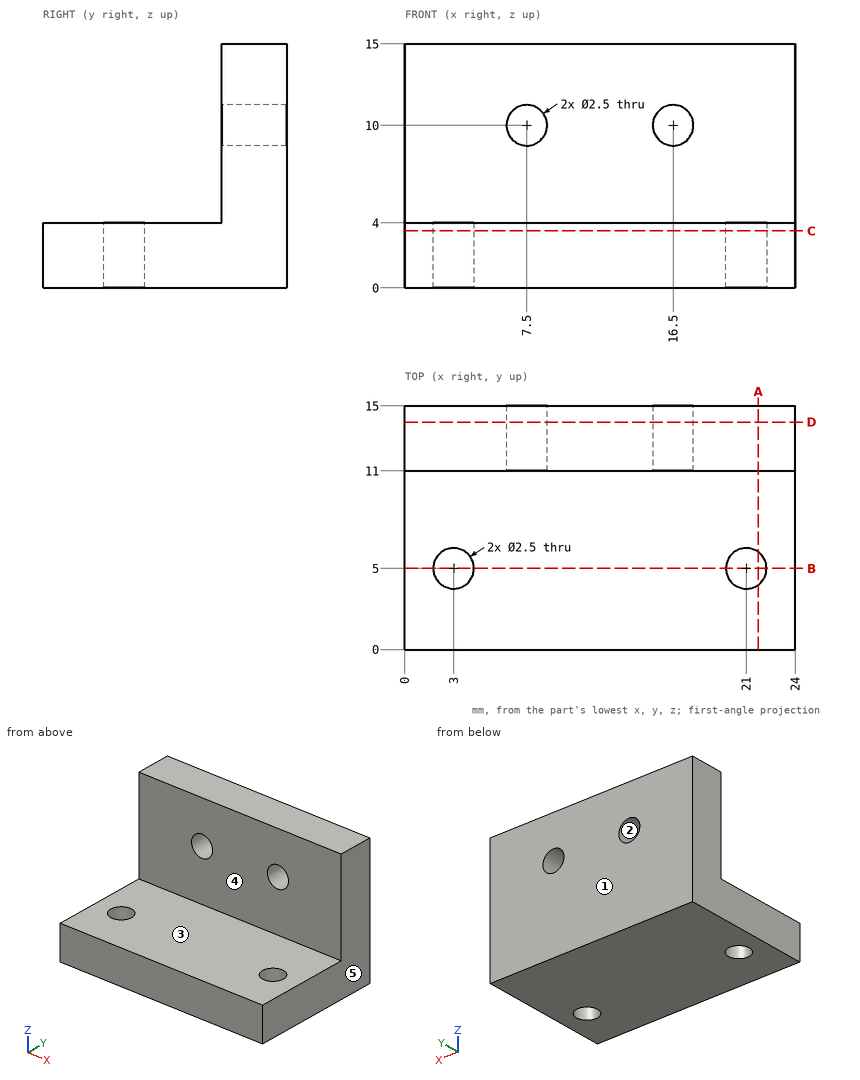
Answer from the drawing. Dimensions are ordinates in mm from the lowest x, y and z of the part. A direction names the side the tool comes from. Round coordinates to 2 decimals unless told otherwise and drop trailing zeros. Loops run counter-clockwise (first coordinate to the right, second up) from the corner with the lowest first, then second, coordinate; pieces in that order, holes last. Notation, with made-up numbers: (36.25, -24) - (68.25, -24) arc R9 ccw to (68.25, -19) - close; hole circle Ø9 at (68, 83). An arc over 180 degrees is marked (long way). Return JSON: item names as keys, results as strings. Group by question number.
1. The part is cut by section D-D on y = 14. Determine the outline of the cut face in (x, z).
2. The part is cut by section B-B on y = 5. Determine the outline of the cut face in (x, z), then the cut area to 3 significant figures.
3. Consider probe 1 along Z at (x, y) = (16.5, 13.4); probe 2 along Y at (x, z) = (21, 2.9); probe 3 along Y at (x, z) = (7.25, 7.5). Determine where each line is inside the solid, lowest interval first.
4. The part is cut by section C-C on z = 3.5. Determine the outline of the cut face in (x, y).
5. The part is cut by section A-A on x = 21.75. Determine the outline of the cut face in (y, z), then the cut area to 3 significant figures.
6. Which of the six approach directions +Z, -Z, +X, -X, +Y, -Y give full straight-line access (tool end or side, diameter ignored) to the marked faces 4 and 5?
7. Each of these flat-tipped pins is pushed along its axis until it touches: P1, Ø5.5, axis at x = 14.5, y = 4.5, coming from the +Z side; P2, Ø4, axis at x = 16.5, z = 10, coming from the -Y side. Where does it stop, or does it pass through?
8. The mould has two halves that part along Z. Classify the marked faces 1, 2 and 3: pulls with the +Z half, pulls with the -Z half, needs draft (parallel to the pull), parting line crosses it, or undercut.
Resolved:
{
 "1": {"outline": "(0, 0) - (24, 0) - (24, 15) - (0, 15) - close; hole circle Ø2.5 at (7.5, 10); hole circle Ø2.5 at (16.5, 10)"},
 "2": {"outline": "(0, 0) - (1.75, 0) - (1.75, 4) - (0, 4) - close; (4.25, 0) - (19.75, 0) - (19.75, 4) - (4.25, 4) - close; (22.25, 0) - (24, 0) - (24, 4) - (22.25, 4) - close", "area": "76.0 mm²"},
 "3": {"probe 1": "z = 0 to 8.75, 11.25 to 15", "probe 2": "y = 0 to 3.75, 6.25 to 15", "probe 3": "y = 11 to 15"},
 "4": {"outline": "(0, 0) - (24, 0) - (24, 15) - (0, 15) - close; hole circle Ø2.5 at (3, 5); hole circle Ø2.5 at (21, 5)"},
 "5": {"outline": "(0, 0) - (4, 0) - (4, 4) - (0, 4) - close; (6, 0) - (15, 0) - (15, 15) - (11, 15) - (11, 4) - (6, 4) - close", "area": "96.0 mm²"},
 "6": {"face 4": "+Z, +X, -X, -Y", "face 5": "+Z, -Z, +X, +Y, -Y"},
 "7": {"P1": "stops at z = 4", "P2": "stops at y = 11"},
 "8": {"face 1": "needs draft", "face 2": "undercut", "face 3": "pulls with the +Z half"}
}
